Study the drawing (mm; zero at the part's minimum x, y, z) and answer. A direction names the side the tool comes from. Coordinates: 2 decimals unless noted, no trailing zeros. Write each loop counter-clockwise with the first axis right and the second up, starting at its lowest first coordinate (ties: lowest second). Pieces come first, ordered by that corner, then holes. Notation, with made-up numbers: M 42,-10.5 L 56,-10.5 A36 ccw 56,26.5 Z; hole C 59,83.5 d6. An arc over 180 degrees is marked long. Answer as CSV lines item,"result". Start each with the question number.
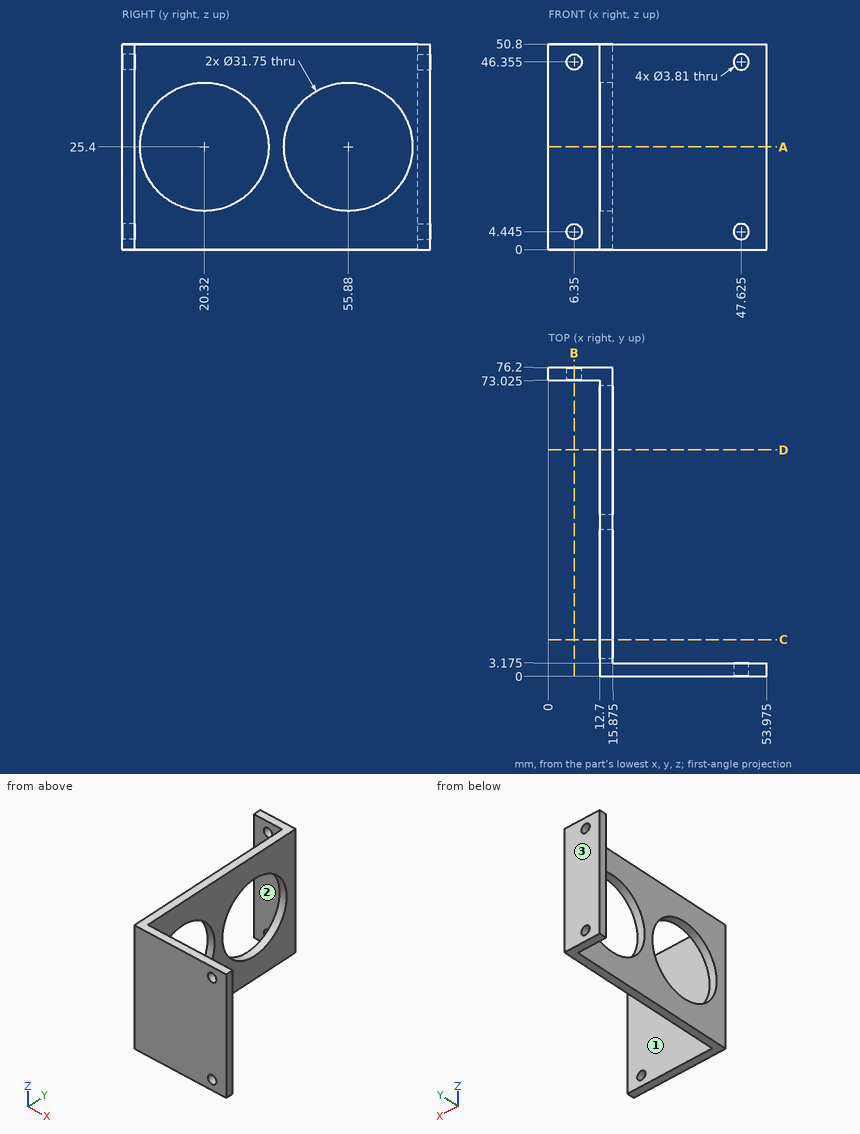
1) The part is cut by section B-B (x = 6.35). Determine the outline of the cut face in (y, z) (3 decimals), then the cut area to 3 significant figures.
2) The part is cut by section A-A (z = 25.4). Determine the outline of the cut face in (x, y) (3 decimals), then the cut area to 3 significant figures.
3) The part is cut by section D-D (y = 55.88). Determine the outline of the cut face in (x, z) (3 decimals), then the cut area to 3 significant figures.
4) Find the intervals of material crossed by line 1 (Y direction, x = 48.5, z = 20) (3 decimals); line 2 (Z direction, x = 14.3, y = 20.32) (3 decimals); line 3 (Z direction, x = 14.5, y = 53.5), in increasing order. Write a range as from..to.
5) Which of the six approach directions +Z, -Z, +X, -X, +Y, -Y give full straight-line access (tool end or side, diameter ignored) to the marked faces 1, 2 and 3?
6) Each of these flat-tipped pins is pushed along its axis until it touches: P1, Ø3, axis at y = 66, z = 15, coming from the -X side; P2, Ø2, axis at x = 17, z = 12.5, coming from the +Y side (3 decimals); P3, Ø1, axis at y = 55, z = 7, coming from the +X side (3 decimals); P4, Ø4.5, axis at x = 47.625, z = 46.355, coming from the -Y side. Where does it stop, or does it pass through?
7) The part is cut by section C-C (y = 9). Determine the outline of the cut face in (x, z) (3 decimals), then the cut area to 3 significant figures.
Completed:
1,outline,"M 73.025,0 L 76.2,0 L 76.2,2.54 L 73.025,2.54 Z; M 73.025,6.35 L 76.2,6.35 L 76.2,44.45 L 73.025,44.45 Z; M 73.025,48.26 L 76.2,48.26 L 76.2,50.8 L 73.025,50.8 Z"
1,area,"137 mm²"
2,outline,"M 0,73.025 L 12.7,73.025 L 12.7,71.755 L 15.875,71.755 L 15.875,76.2 L 0,76.2 Z; M 12.7,0 L 53.975,0 L 53.975,3.175 L 15.875,3.175 L 15.875,4.445 L 12.7,4.445 Z; M 12.7,36.195 L 15.875,36.195 L 15.875,40.005 L 12.7,40.005 Z"
2,area,"202 mm²"
3,outline,"M 12.7,0 L 15.875,0 L 15.875,9.525 L 12.7,9.525 Z; M 12.7,41.275 L 15.875,41.275 L 15.875,50.8 L 12.7,50.8 Z"
3,area,"60.5 mm²"
4,line 1,"0..3.175"
4,line 2,"0..9.525, 41.275..50.8"
4,line 3,"0..9.7, 41.1..50.8"
5,face 1,"+Z, -Z, +X, +Y"
5,face 2,"+Z, -Z, -X, -Y"
5,face 3,"+Z, -Z, +X, -X, +Y"
6,P1,"x = 12.7"
6,P2,"y = 3.175"
6,P3,"x = 15.875"
6,P4,"y = 0"
7,outline,"M 12.7,0 L 15.875,0 L 15.875,14.27 L 12.7,14.27 Z; M 12.7,36.53 L 15.875,36.53 L 15.875,50.8 L 12.7,50.8 Z"
7,area,"90.6 mm²"
